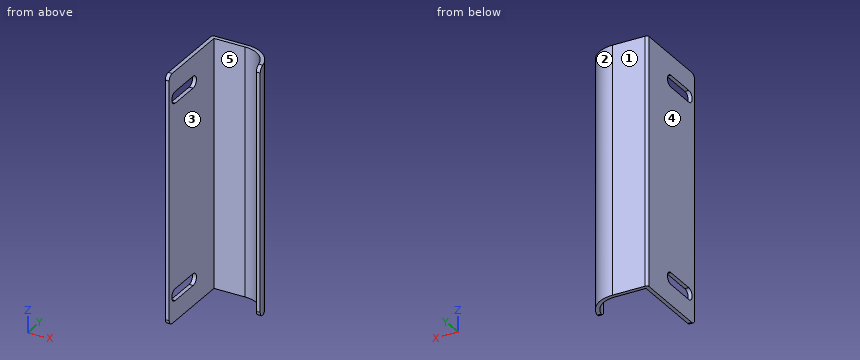
from build123d import *

# Parameters (mm, degrees)
BOSS_EXTRUDE1_DEPTH = 95
FILLET1_R           = 1
FILLET2_R           = 2
CUT_EXTRUDE1_DEPTH  = 2.5


with BuildPart() as part:
    # Sketch1 → Boss-Extrude1 (new body)
    with BuildSketch(Plane.XY):
        with BuildLine():
            Line((-9.763392857, -19.416294643), (-9.763392857, 12.083705357))
            Line((-9.763392857, 12.083705357), (3.736607143, 12.083705357))
            ThreePointArc((3.736607143, 12.083705357), (11.868335127, 8.715433341), (15.236607143, 0.583705357))
            Line((15.236607143, 0.583705357), (13.736607143, 0.583705357))
            ThreePointArc((13.736607143, 0.583705357), (10.807674955, 7.654773169), (3.736607143, 10.583705357))
            Line((3.736607143, 10.583705357), (-8.263392857, 10.583705357))
            Line((-8.263392857, 10.583705357), (-8.263392857, -19.416294643))
            Line((-8.263392857, -19.416294643), (-9.763392857, -19.416294643))
        make_face()
    extrude(amount=BOSS_EXTRUDE1_DEPTH)

    # Fillet1
    fillet1_edges = [part.edges().sort_by_distance(p)[0] for p in [
        (-9.763392857, 12.083705357, 47.5),
    ]]
    fillet(fillet1_edges, radius=FILLET1_R)

    # Fillet2
    fillet2_edges = [part.edges().sort_by_distance(p)[0] for p in [
        (-9.013392857, -19.416294643, 0),
        (14.486607143, 0.583705357, 95),
        (-9.013392857, -19.416294643, 95),
        (14.486607143, 0.583705357, 0),
    ]]
    fillet(fillet2_edges, radius=FILLET2_R)

    # Sketch2 → Cut-Extrude1 (cut, through all)
    with BuildSketch(Plane(origin=(-8.263392857, 0, 0), x_dir=(0, 0, -1), z_dir=(1, 0, 0))):
        with BuildLine():
            Line((-87.25, -3.416294643), (-87.25, -15.416294643))
            ThreePointArc((-87.25, -15.416294643), (-85, -17.666294643), (-82.75, -15.416294643))
            Line((-82.75, -15.416294643), (-82.75, -3.416294643))
            ThreePointArc((-82.75, -3.416294643), (-85, -1.166294643), (-87.25, -3.416294643))
        make_face()
        with BuildLine():
            Line((-12.25, -3.416294643), (-12.25, -15.416294643))
            ThreePointArc((-12.25, -15.416294643), (-10, -17.666294643), (-7.75, -15.416294643))
            Line((-7.75, -15.416294643), (-7.75, -3.416294643))
            ThreePointArc((-7.75, -3.416294643), (-10, -1.166294643), (-12.25, -3.416294643))
        make_face()
    extrude(amount=-CUT_EXTRUDE1_DEPTH, mode=Mode.SUBTRACT)


solid = part.part
The listing builds one solid part. Answer for the finished solid, in the listing's coordinates (mm). Face numbers are marked on the shaded views. A direction names the side the tool comes from. Round coordinates to 2 decimals unless told otherwise and drop trailing zeros. Order: outer loops, then holes, each group sorted by start corner. A loop starts at its lowest first (then second) coordinate and runs counter-clockwise, first axis right, second up. Notation, with made-up numbers: (29.5, 47.25) -> (57.5, 47.25) arc R23 ccw to (57.5, 84.25) -> close; hole circle Ø6 at (20.5, 36.5). An arc over 180 degrees is marked (long way). Put each result on its own line as item: value.
Q1. Section C-C, the plane z = 22.5 is taken. Write down the section's boundary in (x, y).
Results list:
outline: (-9.76, -19.42) -> (-8.26, -19.42) -> (-8.26, 10.58) -> (3.74, 10.58) arc R10 cw to (13.74, 0.58) -> (15.24, 0.58) arc R11.5 ccw to (3.74, 12.08) -> (-8.76, 12.08) arc R1 ccw to (-9.76, 11.08) -> close
Q2. Section A-A, the plane z = 85 is taken. Write down the section's boundary in (x, y).
Results list:
outline: (-9.76, -19.42) -> (-8.26, -19.42) -> (-8.26, -17.67) -> (-9.76, -17.67) -> close; (-9.76, -1.17) -> (-8.26, -1.17) -> (-8.26, 10.58) -> (3.74, 10.58) arc R10 cw to (13.74, 0.58) -> (15.24, 0.58) arc R11.5 ccw to (3.74, 12.08) -> (-8.76, 12.08) arc R1 ccw to (-9.76, 11.08) -> close
Q3. Consider line 1 along X through (y, z) = (1, 78); line 2 along X through (y, z) = (2.5, 74); line 3 along X through (y, z) = (0, 65). Determine where each line is inside the solid, lowest interval first.
Results list:
line 1: -9.76 to -8.26, 13.73 to 15.23
line 2: -9.76 to -8.26, 13.55 to 15.08
line 3: -9.76 to -8.26
Q4. Each of these flat-tipped pins is pushed along its axis until it touches: P1, Ø2, axis at y = 3, z = 37.5, coming from the +X side; P2, Ø8, axis at x = -3, y = -6, coming from the +Z side; P3, Ø3.5, axis at x = 0.5, z = 33.5, coming from the -Y side; P4, Ø1.2, axis at x = 15, z = 47.5, coming from the -Y side. Where does it stop, or does it pass through?
Results list:
P1: x = 15.15
P2: through
P3: y = 10.58
P4: y = 0.58
Q5. Which of the six approach directions +Z, -Z, +X, -X, +Y, -Y give full straight-line access (tool end or side, diameter ignored) to the marked faces 4 and 5?
Results list:
face 4: +Z, -Z, -X, +Y, -Y
face 5: +Z, -Z, -Y
Q6. Section B-B, the plane y = 6 is taken. Write down the section's boundary in (x, z), and give its area (3 significant figures).
Results list:
outline: (-9.76, 0) -> (-8.26, 0) -> (-8.26, 95) -> (-9.76, 95) -> close; (12.14, 0) -> (13.88, 0) -> (13.88, 95) -> (12.14, 95) -> close
area: 308 mm^2
Q7. Section D-D, the plane x = -4.5 is taken. Write down the section's boundary in (y, z).
Results list:
outline: (10.58, 0) -> (12.08, 0) -> (12.08, 95) -> (10.58, 95) -> close
Q8. Determine the mould class of the marked faces 1, 2 and 3 for opening direction X: pulls with the +X half, pulls with the -X half, needs draft (parallel to the pull), parting line crosses it, or undercut.
Results list:
face 1: needs draft
face 2: pulls with the +X half
face 3: undercut
